For this review, take the finished solid that the model builds, in its own axes (mm). A direction names the side the tool comes from. Coordinates: 2 decimals unless noted, no trailing zeros. Write each loop counter-clockwise with the first axis right and the second up, starting at its lowest first coordinate (ties: lowest second). Pieces come first, ordered by that corner, then holes. Notation, with made-up numbers: M 13.5,57 L 25.5,57 A28 ccw 25.5,77 Z; hole C 12.25,-14.75 d4. An arc over 180 degrees is marked long. Return JSON: item names as keys, results as strings.
Autodesk Inventor part; units mm, degrees
ref_plane "YZ Plane" through (0, 0, 0) normal (1, 0, 0) x (0, 1, 0)
ref_plane "XZ Plane" through (0, 0, 0) normal (0, 1, 0) x (-1, 0, 0)
ref_plane "XY Plane" through (0, 0, 0) normal (0, 0, 1) x (1, 0, 0)
sketch "Náčrt2" plane through (0, 0, 0) normal (0, 1, 0) x (-1, 0, 0)
  line L0 (11.5, 17.5) -> (-11.5, 17.5) construction
  line L1 (-17.5, 11.5) -> (-17.5, -11.5) construction
  line L2 (-11.5, -17.5) -> (11.5, -17.5) construction
  line L3 (17.5, -11.5) -> (17.5, 11.5) construction
  line L4 (42.5, 36) -> (42.5, -77.5)
  line L5 (9, -22.5) -> (-14, -22.5) construction
  line L6 (-20, -28.5) -> (-20, -51.5) construction
  line L7 (-14, -57.5) -> (9, -57.5) construction
  line L8 (15, -51.5) -> (15, -28.5) construction
  arc A0 (15, -28.5) -> (9, -22.5) centre (9, -28.5) ccw construction
  arc A1 (9, -57.5) -> (15, -51.5) centre (9, -51.5) ccw construction
  arc A2 (-20, -51.5) -> (-14, -57.5) centre (-14, -51.5) ccw construction
  arc A3 (-14, -22.5) -> (-20, -28.5) centre (-14, -28.5) ccw construction
  line L9 (-45.6938, -20) -> (9, -20) construction
  arc A4 (17.5, -28.5) -> (9, -20) centre (9, -28.5) ccw construction
  line L10 (17.5, -28.5) -> (17.5, -51.5) construction
  line L11 (17.5, -51.5) -> (15, -51.5) construction
  line L12 (-14, -22.5) -> (-45.6938, -22.5) construction
  line L13 (-45.6938, -22.5) -> (-45.6938, -20) construction
  arc A5 (17.5, 11.5) -> (11.5, 17.5) centre (11.5, 11.5) ccw construction
  arc A6 (11.5, -17.5) -> (17.5, -11.5) centre (11.5, -11.5) ccw construction
  arc A7 (-17.5, -11.5) -> (-11.5, -17.5) centre (-11.5, -11.5) ccw construction
  arc A8 (-11.5, 17.5) -> (-17.5, 11.5) centre (-11.5, 11.5) ccw construction
  line L14 (-11.5, -20) -> (11.5, -20) construction
  line L15 (-20, 73.4113) -> (-20, -11.5) construction
  arc A9 (-20, -11.5) -> (-11.5, -20) centre (-11.5, -11.5) ccw construction
  line L16 (-17.5, 11.5) -> (-17.5, 73.4113) construction
  line L17 (-17.5, 73.4113) -> (-20, 73.4113) construction
  line L18 (11.5, -20) -> (11.5, -17.5) construction
  line L19 (17.5, 17.5) -> (-17.5, 17.5) construction
  line L20 (-17.5, 17.5) -> (-17.5, 52.5) construction
  line L21 (-17.5, 52.5) -> (17.5, 52.5) construction
  line L22 (17.5, 52.5) -> (17.5, 17.5) construction
  circle A10 centre (0, 35) radius 6.5
  arc A11 (0, 51) -> (0, 19) centre (0, 35) ccw
  line L23 (0, 51) -> (27.5, 51)
  line L24 (0, 19) -> (11.5, 19)
  line L25 (27.5, 51) -> (42.5, 36)
  arc A12 (17.5, 13) -> (11.5, 19) centre (11.5, 13) ccw
  line L26 (17.5, 13) -> (17.5, -51.5)
  line L27 (-13.5, -57.5) -> (-13.5, -59.2574)
  line L28 (-12.6213, -61.3787) -> (14.1066, -88.1066)
  line L29 (24.7132, -92.5) -> (27.5, -92.5)
  arc A13 (27.5, -92.5) -> (42.5, -77.5) centre (27.5, -77.5) ccw
  arc A14 (14.1066, -88.1066) -> (24.7132, -92.5) centre (24.7132, -77.5) ccw
  arc A15 (-13.5, -59.2574) -> (-12.6213, -61.3787) centre (-10.5, -59.2574) ccw
  line L30 (17.5, -51.5) -> (17.5, -51.5)
  line L31 (6.4677, -58.2408) -> (-10.5, -57.5)
  line L32 (-13.5, -57.5) -> (-10.5, -57.5)
  line L33 (6.4677, -58.2408) -> (6.5, -57.5)
  line L34 (6.5, -57.5) -> (11.5, -57.5)
  arc A16 (11.5, -57.5) -> (17.5, -51.5) centre (11.5, -51.5) ccw
  point P0 (0, 0)
  point P1 (17.5, 0)
  point P2 (0, 17.5)
  point P3 (42.5, 51)
  point P4 (17.5, 35)
  point P5 (0, 52.5)
  point P6 (-13.5, -60.5)
  dimension "d34" = 35
  dimension "d35" = 6
  dimension "d36" = 5
  dimension "d37" = 2.5
  dimension "d38" = 2.5
  dimension "d39" = 6
  dimension "d40" = 2.5
  dimension "d43" = 25
  dimension "d46" = 13
  dimension "d47" = 32
  dimension "d48" = 15
  dimension "d49" = 15
  dimension "d50" = 6
  dimension "d51" = 35
  dimension "d55" = 3
  dimension "d56" = 15
  dimension "d57" = 15
  dimension "d58" = 3
  dimension "d60" = 35
  dimension "d61" = 3
  dimension "d62" = 2.5
  dimension "d63" = 35
  dimension "d64" = 45
  dimension "d66" = 31
  dimension "d69" = 6
  dimension "d72" = 2.5
extrude "Vysunutí1" add sketch "Náčrt2" along normal blind 6
fillet "Zaoblení3" radius 2 1 edges at (13.5, 3, -57.5)
fillet "Zaoblení4" radius 10 2 edges at (-27.5, 3, 51) (-42.5, 3, 36)
fillet "Zaoblení5" radius 1 2 edges at (-6.5, 3, -57.5) (-6.4677, 3, -58.2408)
equation "\"PoloměrOhybu\" = Tloušťka"
equation "\"ŠířkaVýštipu\" = Tloušťka"
equation "\"HloubkaVýštipu\" = 0.5 * Tloušťka"
equation "\"VelikostRohovéhoVýštipu\" = 4 * Tloušťka"
equation "\"MinimálníZbytek\" = 2 * Tloušťka"
equation "\"PřechodovýPoloměr\" = PoloměrOhybu"
equation "\"VelikostJacobihoPoloměru\" = PoloměrOhybu"
equation "\"VelikostMezery\" = Tloušťka"
properties part number "DD_KVD_002_07" material "Nerezová ocel"
1. For faces 5 (the face through (-15.696, 2.958, 17.289)), 6 (the face through (-41.76, 3.04, 35.63)), 7 (the face through (2.387, 2.958, -57.854)), list the 3-axis set-ups (+Z, -Z, +X, -X, +Y, -Y) from which the entire face can be reached by the end or side of a thin tool; tool diameter is ignored.
Checks:
{"face 5": "+X, +Y, -Y", "face 6": "+Z, -X, +Y, -Y", "face 7": "+Y, -Y"}
2. We need section C-C (z = -2.5). State the section outline as (x, y) points, plus the area to 3 significant figures.
Checks:
{"outline": "M -42.5,0 L -17.5,0 L -17.5,6 L -42.5,6 Z", "area": "150 mm2"}
3. We need section D-D (z = 16). State the section outline as (x, y) points.
Checks:
{"outline": "M -42.5,0 L -16.7,0 L -16.7,6 L -42.5,6 Z"}
4. We need section A-A (z = 35). State the section outline as (x, y) points, plus the area to 3 significant figures.
Checks:
{"outline": "M -41.99,0 L -6.5,0 L -6.5,6 L -41.99,6 Z; M 6.5,0 L 16,0 L 16,6 L 6.5,6 Z", "area": "270 mm2"}
5. Clearance check with flat-ended pins moving along their axes: pin 1 Ø1.8 at (x, y) = (-8, 2) entering from -Z; pin 2 Ø3 at (x, y) = (4.5, 4) entering from -Z; pin 3 Ø1.8 at (y, z) = (1.5, -6.5) entering from +X. State where each tip first meets the part, or that it passes through.
Checks:
{"pin 1": "z = -82.9", "pin 2": "z = -71", "pin 3": "x = -17.5"}
6. Wall thickness on L1, parallel to Z at x = 0, y = 4.25; L2, parallel to Z at x = 6, y = 4.5; L3, parallel to X at y = 5.75, z = -52: over which ranges is each line inside the solid? List them lowest first. Write a range as from..to.
Checks:
{"L1": "-74..-57.96, 19..28.5, 41.5..51", "L2": "-68..-57.7, 20.17..32.5, 37.5..49.83", "L3": "-42.5..-17.48"}
7. Draft analysis for pull direction Z (two halves, no side actions). For faces 1 (the face through (-26, 3, -92.5)), 2 (the face through (-27.235, 3.042, 50.218)), 3 (the face through (-19, 6, -20)), 4 (the face through (-9, 3, -57.5)), state which applies: +Z half, -Z half, draft (parallel to the pull), parting line (faces both ways), or undercut.
Checks:
{"face 1": "-Z half", "face 2": "+Z half", "face 3": "draft", "face 4": "undercut"}
8. We need section B-B (x = 2). State the section outline as (y, z) points, plus the area to 3 significant figures.
Checks:
{"outline": "M 0,-72 L 6,-72 L 6,-57.87 L 0,-57.87 Z; M 0,19.13 L 6,19.13 L 6,28.82 L 0,28.82 Z; M 0,41.18 L 6,41.18 L 6,50.87 L 0,50.87 Z", "area": "201 mm2"}
